Input: part model. Units: mm. Frame: model coordinates. Round coordinates to 2 decimals unless told otherwise and drop trailing zeros. Write each loop counter-clockwise with the first axis right and the second up, starting at its lowest first coordinate (ties: lowest second). Pieces come first, ordered by that corner, then holes. Notation, with made-up numbers: M 79,15 L 119,15 A26 ccw 119,44 Z; hole C -35,6 d9. An arc over 180 degrees is marked long. Answer as CSV lines item,"result". Start each with the question number.
```python
from build123d import *

# Parameters (mm, degrees)
SKETCH1_W           = 76.2
SKETCH1_H           = 4.7625
BOSS_EXTRUDE1_DEPTH = 508
CUT_EXTRUDE1_DEPTH  = 5.7625
SKETCH3_R           = 2.0828
CUT_EXTRUDE2_DEPTH  = 5.7625


with BuildPart() as part:
    # Sketch1 → Boss-Extrude1 (new body)
    with BuildSketch(Plane.XY):
        with Locations((0, 20.514000599)):
            Rectangle(SKETCH1_W, SKETCH1_H)
    extrude(amount=BOSS_EXTRUDE1_DEPTH)

    # Sketch2 → Cut-Extrude1 (cut, through all)
    with BuildSketch(Plane(origin=(0, 22.895250599, 0), x_dir=(1, 0, 0), z_dir=(0, 1, 0))):
        with BuildLine():
            Line((-19.05, -184.15), (-38.1, -184.15))
            Line((-38.1, -184.15), (-38.1, -222.25))
            Line((-38.1, -222.25), (-19.05, -222.25))
            ThreePointArc((-19.05, -222.25), (0, -203.2), (-19.05, -184.15))
        make_face()
        with BuildLine():
            Line((19.05, -323.85), (38.1, -323.85))
            Line((38.1, -323.85), (38.1, -285.75))
            Line((38.1, -285.75), (19.05, -285.75))
            ThreePointArc((19.05, -285.75), (0, -304.8), (19.05, -323.85))
        make_face()
    extrude(amount=-CUT_EXTRUDE1_DEPTH, mode=Mode.SUBTRACT)

    # Sketch3 → Cut-Extrude2 (cut, through all)
    with BuildSketch(Plane(origin=(0, 22.895250599, 0), x_dir=(1, 0, 0), z_dir=(0, 1, 0))):
        with Locations((-31.75, -488.95)):
            Circle(SKETCH3_R)
        with Locations((31.75, -19.05)):
            Circle(SKETCH3_R)
    cut_extrude2 = extrude(amount=-CUT_EXTRUDE2_DEPTH, mode=Mode.SUBTRACT)

    # Mirror1: Cut-Extrude2 across plane
    add(cut_extrude2.mirror(Plane.XY.offset(254)), mode=Mode.SUBTRACT)


solid = part.part
```
Item 1: Cut plane A-A, the plane y = 19.15. Return loops of the section in (x, z).
Item 2: Draft query along Z for faces 1 (the face through (-1, 22.895, 250)), 2 (the face through (-0.005, 20.547, 203.619)). Return one class per face: +Z half, -Z half, draft (parallel to the pull), parting line (faces both ways), or undercut.
Item 3: Cut plane B-B, the plane x = 9.5. Return loops of the section in (y, z), plus the area to 3 significant figures.
Item 4: Cut plane C-C, the plane x = -12. Return loops of the section in (y, z).
Item 5: Line query: line 1 (Z direction, x = -31.75, y = 19.6); line 2 (X direction, y = 21.9, z = 488.95); line 3 (Z direction, x = -34.5, y = 22.5). Output: solid intervals per line, ascending. Write a range as [from, to].
Results list:
1,outline,"M -38.1,0 L 38.1,0 L 38.1,285.75 L 19.05,285.75 A19.05 cw 19.05,323.85 L 38.1,323.85 L 38.1,508 L -38.1,508 L -38.1,222.25 L -19.05,222.25 A19.05 cw -19.05,184.15 L -38.1,184.15 Z; hole C -31.75,19.05 d4.17; hole C -31.75,488.95 d4.17; hole C 31.75,19.05 d4.17; hole C 31.75,488.95 d4.17"
2,face 1,"draft"
2,face 2,"undercut"
3,outline,"M 18.13,0 L 22.9,0 L 22.9,288.32 L 18.13,288.32 Z; M 18.13,321.28 L 22.9,321.28 L 22.9,508 L 18.13,508 Z"
3,area,"2,260 mm²"
4,outline,"M 18.13,0 L 22.9,0 L 22.9,185.5 L 18.13,185.5 Z; M 18.13,220.9 L 22.9,220.9 L 22.9,508 L 18.13,508 Z"
5,line 1,"[0, 16.97], [21.13, 184.15], [222.25, 486.87], [491.03, 508]"
5,line 2,"[-38.1, -33.83], [-29.67, 29.67], [33.83, 38.1]"
5,line 3,"[0, 184.15], [222.25, 508]"
